Read the model definition and answer for the solid it produces. Units are mm, in the model's axes. Face numbers are marked on the shaded views. Coordinates: 2 decimals unless noted, no trailing zeros. Loops run counter-clockwise (first coordinate to the right, second up) from the corner with the lowest first, then second, coordinate; pieces in that order, holes last.
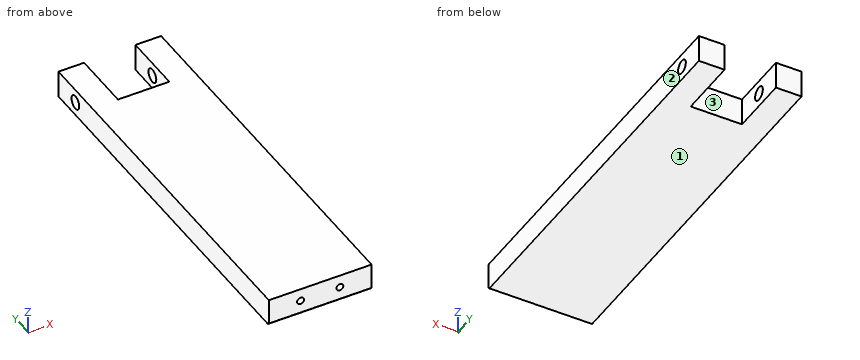
from build123d import *

# Parameters (mm, degrees)
SKETCH1_W               = 60
SKETCH1_H               = 250
BOSS_EXTRUDE1_DEPTH     = 16
CHAMFER1_SIZE           = 1
SKETCH2_R               = 2
CUT_EXTRUDE1_DEPTH      = 15
CUT_EXTRUDE4_REACH      = 259.597
SKETCH5_W               = 30
SKETCH5_H               = 35
CUT_EXTRUDE5_DEPTH      = 255.521118967
CUT_EXTRUDE5_DEPTH_BACK = 255.521118967
SKETCH6_R               = 4
SKETCH7_W               = 60
SKETCH7_H               = 32.5
CUT_EXTRUDE6_DEPTH      = 258.596583828


with BuildPart() as part:
    # Sketch1 → Boss-Extrude1 (new body)
    with BuildSketch(Plane.XY):
        with Locations((30, 125)):
            Rectangle(SKETCH1_W, SKETCH1_H)
    extrude(amount=BOSS_EXTRUDE1_DEPTH)

    # Chamfer1
    chamfer1_edges = [part.edges().sort_by_distance(p)[0] for p in [
        (30, 0, 0),
    ]]
    chamfer(chamfer1_edges, length=CHAMFER1_SIZE)

    # Sketch2 → Cut-Extrude1 (cut)
    with BuildSketch(Plane(origin=(0, 0, 0), x_dir=(-1, 0, 0), z_dir=(0, -1, 0))):
        with Locations(Location((-41.5, -8.5, 0), (0, 0, 90))):
            Circle(SKETCH2_R)
        with Locations(Location((-18.5, -8.5, 0), (0, 0, 90))):
            Circle(SKETCH2_R)
    extrude(amount=-CUT_EXTRUDE1_DEPTH, mode=Mode.SUBTRACT)

    # Sketch5 → Cut-Extrude4 (cut, up to next)
    with BuildSketch(Plane(origin=(0, 0, 0), x_dir=(-1, 0, 0), z_dir=(0, 0, -1)), mode=Mode.PRIVATE) as cut_extrude4_sk1:
        with Locations((-30, 200)):
            Rectangle(SKETCH5_W, SKETCH5_H)
    cut_extrude4_tool1 = extrude(cut_extrude4_sk1.sketch, amount=-CUT_EXTRUDE4_REACH, mode=Mode.PRIVATE) & part.part
    add(cut_extrude4_tool1.solids().sort_by_distance((30, 200, 0))[0], mode=Mode.SUBTRACT)

    # Sketch6 → Cut-Extrude5 (cut, two sides: drawn at the far end of the back side and taken through both)
    with BuildSketch(Plane.ZY.offset(-45).offset(-CUT_EXTRUDE5_DEPTH_BACK)):
        with Locations((8, 200)):
            Circle(SKETCH6_R)
    extrude(amount=CUT_EXTRUDE5_DEPTH + CUT_EXTRUDE5_DEPTH_BACK, mode=Mode.SUBTRACT)

    # Sketch7 → Cut-Extrude6 (cut, through all)
    with BuildSketch(Plane(origin=(0, 0, 0), x_dir=(-1, 0, 0), z_dir=(0, 0, -1))):
        with Locations((-30, 233.75)):
            Rectangle(SKETCH7_W, SKETCH7_H)
    extrude(amount=-CUT_EXTRUDE6_DEPTH, mode=Mode.SUBTRACT)


solid = part.part
Q1. Determine the mould class of the marked faces 1, 2 and 3 for opening direction X: +X half, -X half, draft (parallel to the pull), parting line (faces both ways), or undercut.
Findings below:
face 1: draft
face 2: +X half
face 3: undercut
Q2. Straight lines are drawn through the part: probe 1 along X at (y, z) = (11.5, 8.5); probe 2 along X at (y, z) = (207, 5.75); probe 3 along Z at (x, y) = (51.5, 200). For each, find the intervals that lie inside material, in ascending order.
Findings below:
probe 1: x = 0 to 16.5, 20.5 to 39.5, 43.5 to 60
probe 2: x = 0 to 15, 45 to 60
probe 3: z = 0 to 4, 12 to 16
Q3. Flat-ended cylindrical pins translate along their axes: pin 1 Ø2 at (x, z) = (18.5, 8) entering from -Y; pin 2 Ø2.5 at (x, z) = (18.5, 8.5) entering from +Y. Find the tip coordinate at first contact, or state that the pin passes through.
Findings below:
pin 1: stops at y = 15
pin 2: stops at y = 182.5
Q4. A cutting plane is placed at B-B (x = 41.5). Give the vertices of the cut face in (y, z).
Findings below:
outline: (0, 1) - (1, 0) - (182.5, 0) - (182.5, 16) - (0, 16) - (0, 10.5) - (15, 10.5) - (15, 6.5) - (0, 6.5) - close
Q5. A cutting plane is placed at A-A (y = 200). Give the vertices of the cut face in (x, z), then the cut area to 3 significant figures.
Findings below:
outline: (0, 0) - (15, 0) - (15, 4) - (0, 4) - close; (0, 12) - (15, 12) - (15, 16) - (0, 16) - close; (45, 0) - (60, 0) - (60, 4) - (45, 4) - close; (45, 12) - (60, 12) - (60, 16) - (45, 16) - close
area: 240 mm2
Q6. A cutting plane is placed at C-C (z = 8.5). Give the vertices of the cut face in (x, y), then the cut area to 3 significant figures.
Findings below:
outline: (0, 0) - (16.5, 0) - (16.5, 15) - (20.5, 15) - (20.5, 0) - (39.5, 0) - (39.5, 15) - (43.5, 15) - (43.5, 0) - (60, 0) - (60, 196.03) - (45, 196.03) - (45, 182.5) - (15, 182.5) - (15, 196.03) - (0, 196.03) - close; (0, 203.97) - (15, 203.97) - (15, 217.5) - (0, 217.5) - close; (45, 203.97) - (60, 203.97) - (60, 217.5) - (45, 217.5) - close
area: 11,600 mm2
